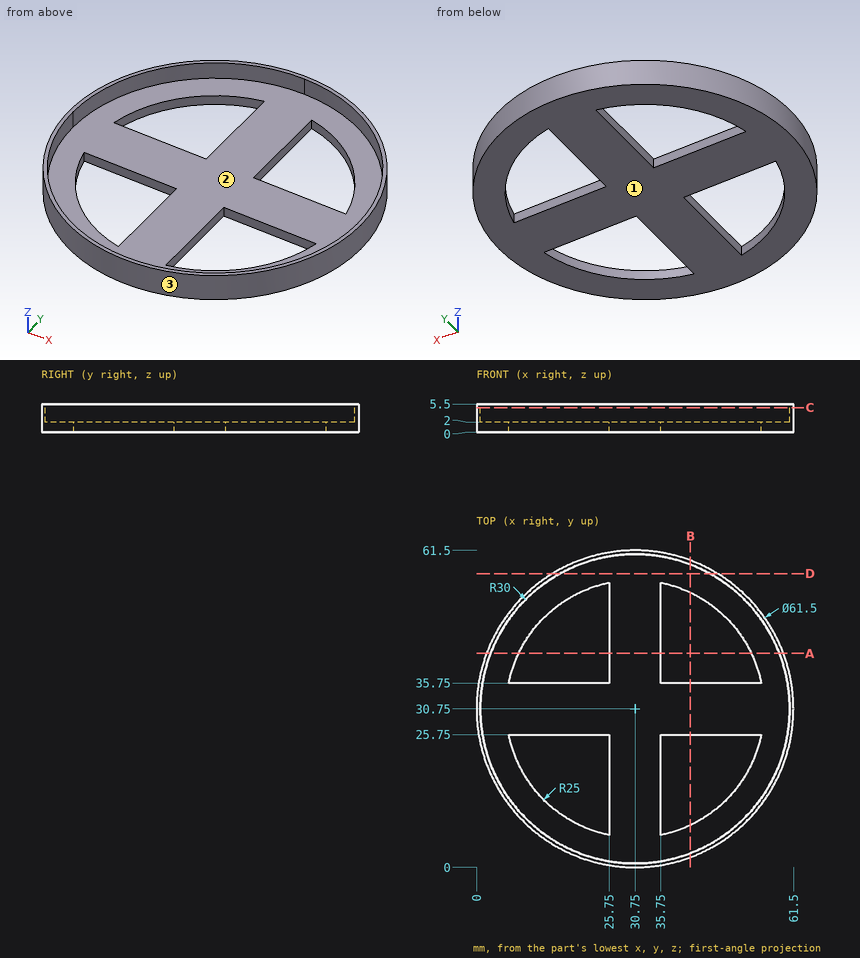
Job drawing, mm, ordinate dimensions from the low corner. One solid piece. Coordinates: 2 decimals unless noted, no trailing zeros. Loops run counter-clockwise (first coordinate to the right, second up) from the corner with the lowest first, then second, coordinate; pieces in that order, holes last. Notation, with made-up numbers: (39.25, 87) - (58.25, 87) arc R24 ccw to (58.25, 107) - close; hole circle Ø3 at (34, 87.5). An arc over 180 degrees is marked (long way). Answer as a JSON object with one key per item and string values. Group by question number.
(1) Cut at A-A (y = 41.5). Give the cut face in (x, z), then the cut area to 3 significant figures.
(2) Two-plate mould, pull along X, no slides. Class the marked faces 1, 2 and 3: released by +X, released by -X, zero draft, split by the parting line, or undercut.
(3) Flat gauge pins, fed straight in: pin 1 (1.5 mm diameter, centred on x = 44, z = 4, fed in from -Y); pin 2 (1 mm diameter, centred on y = 45.5, z = 4, fed in from +X); pin 3 (5 mm diameter, centred on x = 47, y = 22, fed in from -Z); pin 4 (1 mm diameter, centred on y = 11.5, z = 0.5, fed in from +X). Where does each tip first touch, or does it go through?
(4) Probe line 1 along Y through (x, z) = (45.5, 1.1); line 2 along X through (y, z) = (43, 0.4); line 3 along X through (y, z) = (10.5, 1.4). List the from-to ranges inside material, lowest first.
(5) Cut at D-D (y = 57). Give the cut face in (x, z).
(6) Cut at C-C (z = 4.8). Give the cut face in (x, y).
Geometry says:
{
 "1": {"outline": "(1.94, 0) - (8.18, 0) - (8.18, 2) - (2.74, 2) - (2.74, 5.5) - (1.94, 5.5) - close; (25.75, 0) - (35.75, 0) - (35.75, 2) - (25.75, 2) - close; (53.32, 0) - (59.56, 0) - (59.56, 5.5) - (58.76, 5.5) - (58.76, 2) - (53.32, 2) - close", "area": "50.6 mm^2"},
 "2": {"face 1": "zero draft", "face 2": "undercut", "face 3": "split by the parting line"},
 "3": {"pin 1": "stops at y = 2.66", "pin 2": "stops at x = 58", "pin 3": "passes through", "pin 4": "stops at x = 55.12"},
 "4": {"line 1": "y = 3.77 to 10.56, 25.75 to 35.75, 50.94 to 57.73", "line 2": "x = 2.55 to 8.96, 25.75 to 35.75, 52.54 to 58.95", "line 3": "x = 7.61 to 16.09, 25.75 to 35.75, 45.41 to 53.89"},
 "5": {"outline": "(14.73, 0) - (46.77, 0) - (46.77, 5.5) - (45.27, 5.5) - (45.27, 2) - (16.23, 2) - (16.23, 5.5) - (14.73, 5.5) - close"},
 "6": {"outline": "circle Ø61.5 at (30.75, 30.75); hole (0.75, 30.75) arc R30 ccw to (30.75, 0.75) arc R30 ccw to (60.75, 30.75) arc R30 ccw to (30.75, 60.75) arc R30 ccw to start"}
}
